Design review of the part built by this model. Coordinates are the model's own, in mm. Face numbers are marked on the shaded views. A direction names the side the tool comes from. Give positions to 0.01 mm unless a question says otherwise; leave off trailing zeros. Write each loop counter-clockwise with the first axis right and the second up, starting at its lowest first coordinate (ties: lowest second). Pieces come first, ordered by that corner, then holes. Notation, with made-up numbers: (-11.5, 79.5) - (16.5, 79.5) arc R21 cw to (16.5, 97.5) - close; hole circle Ø10 at (-23.75, -24). An arc over 180 degrees is marked (long way). Write each question's results on one line, items separated by ' | '. Start each with the question number.
from build123d import *

# Parameters (mm, degrees)
SKETCH1_W           = 22.75
SKETCH1_H           = 22.45
BOSS_EXTRUDE1_DEPTH = 12.75
SKETCH2_W           = 12.75
SKETCH2_H           = 2.5
BOSS_EXTRUDE2_DEPTH = 4.5
SKETCH3_W           = 12.75
SKETCH3_H           = 2.5
BOSS_EXTRUDE3_DEPTH = 4.5
SKETCH4_R           = 1
CUT_EXTRUDE1_DEPTH  = 2.5
SKETCH5_R           = 1
CUT_EXTRUDE2_DEPTH  = 2.5
SKETCH6_R           = 6.375
BOSS_EXTRUDE4_DEPTH = 4.05
SKETCH7_R           = 2.5
BOSS_EXTRUDE5_DEPTH = 5


with BuildPart() as part:
    # Sketch1 → Boss-Extrude1 (new body)
    with BuildSketch(Plane.XY):
        with Locations((3.479135338, 0)):
            Rectangle(SKETCH1_W, SKETCH1_H)
    extrude(amount=BOSS_EXTRUDE1_DEPTH)

    # Sketch2 → Boss-Extrude2 (add)
    with BuildSketch(Plane(origin=(14.854135338, 0, 0), x_dir=(0, 0, -1), z_dir=(1, 0, 0))):
        with Locations((-6.375, 6.025)):
            Rectangle(SKETCH2_W, SKETCH2_H)
    extrude(amount=BOSS_EXTRUDE2_DEPTH)

    # Sketch3 → Boss-Extrude3 (add)
    with BuildSketch(Plane.ZY.offset(7.895864662)):
        with Locations((6.375, 6.025)):
            Rectangle(SKETCH3_W, SKETCH3_H)
    extrude(amount=BOSS_EXTRUDE3_DEPTH)

    # Sketch4 → Cut-Extrude1 (cut)
    with BuildSketch(Plane(origin=(0, 7.275, 0), x_dir=(1, 0, 0), z_dir=(0, 1, 0))):
        with Locations((-10.145864662, -6.375)):
            Circle(SKETCH4_R)
    extrude(amount=-CUT_EXTRUDE1_DEPTH, mode=Mode.SUBTRACT)

    # Sketch5 → Cut-Extrude2 (cut)
    with BuildSketch(Plane(origin=(0, 7.275, 0), x_dir=(1, 0, 0), z_dir=(0, 1, 0))):
        with Locations((17.104135338, -6.375)):
            Circle(SKETCH5_R)
    extrude(amount=-CUT_EXTRUDE2_DEPTH, mode=Mode.SUBTRACT)

    # Sketch6 → Boss-Extrude4 (add)
    with BuildSketch(Plane(origin=(0, 11.225, 0), x_dir=(1, 0, 0), z_dir=(0, 1, 0))):
        with Locations((-1.520864662, -6.375)):
            Circle(SKETCH6_R)
    extrude(amount=BOSS_EXTRUDE4_DEPTH)

    # Sketch7 → Boss-Extrude5 (add)
    with BuildSketch(Plane(origin=(0, 15.275, 0), x_dir=(1, 0, 0), z_dir=(0, 1, 0))):
        with Locations((-1.520864662, -6.375)):
            Circle(SKETCH7_R)
    extrude(amount=BOSS_EXTRUDE5_DEPTH)


solid = part.part
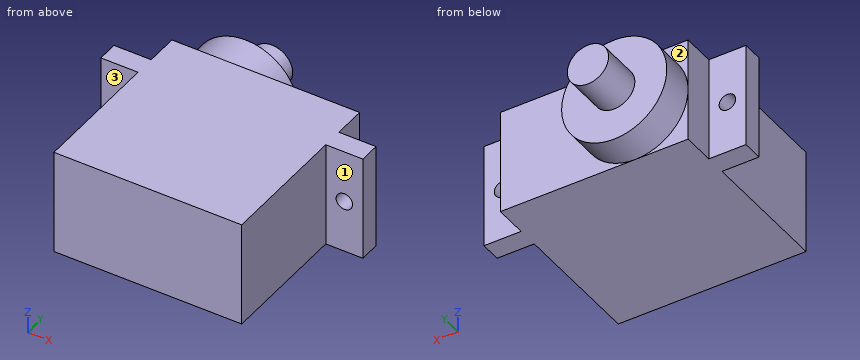
Q1. Add section D-D on y = 0. State the section outline as (x, z) points, plus the area to 3 significant figures.
Q2. Add section B-B on x = -1. State the section outline as (y, z) points (3 decimals).
Q3. Machinability: for the marked faces 1, 2 and 3, which of the approach directions +Z, -Z, +X, -X, +Y, -Y give a long, thin tool a straight path to every point of the face, cutting with its end or side? Answer none if there is none.
Q4. Add section A-A on z = 6.75. State the section outline as (x, y) points (3 decimals), plus the area to 3 significant figures.
Q5. Add section C-C on z = 10.25. State the section outline as (x, y) points (3 decimals), plus the area to 3 significant figures.
Q6. Insertion check: P1, Ø6, axis at y = 17, z = 8, coming from the +X side; P2, Ø5, axis at x = 17.5, z = 8, coming from the +Y side (3 decimals); P3, Ø2, axis at y = 8.5, z = 7.5, coming from the -X side. Each pin has a flat end and moves straight along its axis. Give the tip position at first contact, or say it passes through.
Q7. For line 1 along Y through (x, z) = (2, 10.5) (3 decimals); line 2 along Y through (x, z) = (13, 8.75) (3 decimals); line 3 along X through (y, z) = (-5.5, 4), list the stretches that pass through material, from the lowest coordinate up. Write a range as [from, to].
Result:
1) outline: (-7.9, 0) - (14.85, 0) - (14.85, 12.75) - (-7.9, 12.75) - close | area: 290 mm²
2) outline: (-11.225, 0) - (11.225, 0) - (11.225, 0.021) - (15.275, 0.021) - (15.275, 3.93) - (20.275, 3.93) - (20.275, 8.82) - (15.275, 8.82) - (15.275, 12.729) - (11.225, 12.729) - (11.225, 12.75) - (-11.225, 12.75) - close
3) face 1: +Z, -Z, +X, -Y | face 2: +Z, -X, +Y | face 3: +Z, -Z, -X, -Y
4) outline: (-12.396, 4.775) - (-11.073, 4.775) - (-11.073, 7.275) - (-12.396, 7.275) - close; (-9.219, 4.775) - (-7.896, 4.775) - (-7.896, -11.225) - (14.854, -11.225) - (14.854, 4.775) - (16.177, 4.775) - (16.177, 7.275) - (14.854, 7.275) - (14.854, 11.225) - (4.843, 11.225) - (4.843, 15.275) - (0.951, 15.275) - (0.951, 20.275) - (-3.993, 20.275) - (-3.993, 15.275) - (-7.885, 15.275) - (-7.885, 11.225) - (-7.896, 11.225) - (-7.896, 7.275) - (-9.219, 7.275) - close; (18.031, 4.775) - (19.354, 4.775) - (19.354, 7.275) - (18.031, 7.275) - close | area: 600 mm²
5) outline: (-12.396, 4.775) - (-7.896, 4.775) - (-7.896, -11.225) - (14.854, -11.225) - (14.854, 4.775) - (19.354, 4.775) - (19.354, 7.275) - (14.854, 7.275) - (14.854, 11.225) - (3.541, 11.225) - (3.541, 15.275) - (-6.583, 15.275) - (-6.583, 11.225) - (-7.896, 11.225) - (-7.896, 7.275) - (-12.396, 7.275) - close | area: 574 mm²
6) P1: stops at x = 4.85 | P2: stops at y = 7.275 | P3: stops at x = -7.9
7) line 1: y = [-11.225, 15.275] | line 2: y = [-11.225, 11.225] | line 3: x = [-7.9, 14.85]
